Read the model definition and answer for the solid it produces. Units are mm, in the model's axes. Face numbers are marked on the shaded views. A direction names the side the tool comes from. Coordinates: 2 decimals unless noted, no trailing zeros. Order: outer loops, then holes, each group sorted by start corner. A loop starts at its lowest first (then second) coordinate and runs counter-clockwise, first axis right, second up. Notation, with made-up numbers: (1.25, 5.25) -> (52.25, 5.25) arc R8 ccw to (52.25, 18.25) -> close; hole circle Ø8 at (-11.5, 59). An arc over 180 degrees is marked (long way). Answer in a Markdown table with one row per item.
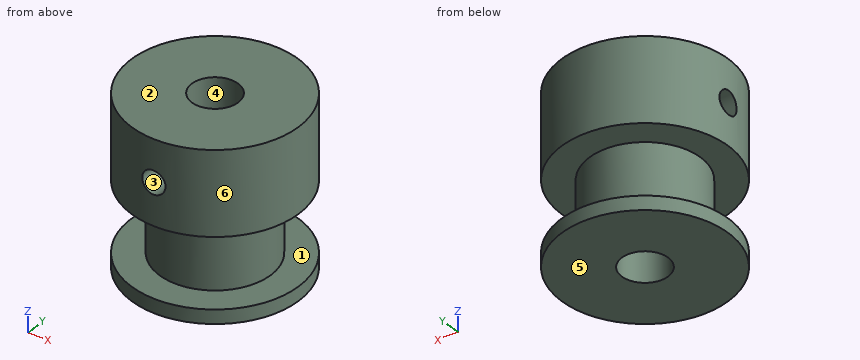
from build123d import *

# Parameters (mm, degrees)
ESQUISSE1_R                  = 9
BOSS_EXTRU_1_DEPTH           = 18
ENL_V_START                  = 1.5
ESQUISSE2_R                  = 9
ESQUISSE2_R_2                = 6
ENL_V_MAT_EXTRU_1_DEPTH      = 7.5
ESQUISSE3_R                  = 2.5
ENL_V_MAT_EXTRU_3_DEPTH      = 23.045407685
ESQUISSE4_R                  = 1.25
ENL_V_MAT_EXTRU_4_DEPTH      = 23.045407685
R_P_TITION_CIRCULAIRE1_COUNT = 2
R_P_TITION_CIRCULAIRE1_ANGLE = 90


with BuildPart() as part:
    # Esquisse1 → Boss.-Extru.1 (new body)
    with BuildSketch(Plane.XY):
        Circle(ESQUISSE1_R)
    extrude(amount=BOSS_EXTRU_1_DEPTH)

    # Esquisse2 → Enlèv. mat.-Extru.1 (cut)
    with BuildSketch(Plane.XY.offset(ENL_V_START)):
        Circle(ESQUISSE2_R)
        Circle(ESQUISSE2_R_2, mode=Mode.SUBTRACT)
    extrude(amount=ENL_V_MAT_EXTRU_1_DEPTH, mode=Mode.SUBTRACT)

    # Esquisse3 → Enlèv. mat.-Extru.3 (cut, through all)
    with BuildSketch(Plane.XY):
        Circle(ESQUISSE3_R)
    extrude(amount=ENL_V_MAT_EXTRU_3_DEPTH, mode=Mode.SUBTRACT)

    # Esquisse4 → Enlèv. mat.-Extru.4 (cut, through all)
    with BuildSketch(Plane(origin=(0, 0, 0), x_dir=(1, 0, 0), z_dir=(0, 1, 0))):
        with Locations(Location((0, -13.5, 0), (0, 0, 270))):
            Circle(ESQUISSE4_R)
    enl_v_mat_extru_4 = extrude(amount=-ENL_V_MAT_EXTRU_4_DEPTH, mode=Mode.SUBTRACT)

    # Répétition circulaire1: Enlèv. mat.-Extru.4 ×2 about axis
    r_p_tition_circulaire1_axis = Axis((0, 0, 18), (0, 0, -1))
    for i in range(1, R_P_TITION_CIRCULAIRE1_COUNT):
        add(enl_v_mat_extru_4.rotate(r_p_tition_circulaire1_axis, i * R_P_TITION_CIRCULAIRE1_ANGLE / (R_P_TITION_CIRCULAIRE1_COUNT - 1)), mode=Mode.SUBTRACT)


solid = part.part
Q1. The part is cut by section D-D (z = 10.5). Write down the section's boundary in (x, y).
Outcome:
| item | result |
|---|---|
| outline | circle Ø18 at (0, 0); hole circle Ø5 at (0, 0) |
Q2. The part is cut by section A-A (x = 0). Write down the section's boundary in (y, z).
Outcome:
| item | result |
|---|---|
| outline | (-9, 0) -> (-2.5, 0) -> (-2.5, 12.25) -> (-9, 12.25) -> (-9, 9) -> (-6, 9) -> (-6, 1.5) -> (-9, 1.5) -> close; (-9, 14.75) -> (-2.5, 14.75) -> (-2.5, 18) -> (-9, 18) -> close; (2.5, 0) -> (9, 0) -> (9, 1.5) -> (6, 1.5) -> (6, 9) -> (9, 9) -> (9, 18) -> (2.5, 18) -> close |
Q3. For the marked faces 1, 2 and 3, determine the directions among +Z, -Z, +X, -X, +Y, -Y from which every point of the face is accessible in a straight line to the end or side of a thin tool.
Outcome:
| item | result |
|---|---|
| face 1 | none |
| face 2 | +Z, +X, -X, +Y, -Y |
| face 3 | -Y |
Q4. For a pull along X with two mould halves and no side action, classify the marked faces 4, 5 and 6 as pulls with the +X half, pulls with the -X half, needs draft (parallel to the pull), parting line crosses it, or undercut.
Outcome:
| item | result |
|---|---|
| face 4 | undercut |
| face 5 | needs draft |
| face 6 | parting line crosses it |
Q5. Given pin 1 (5.5 mm diameter, centred on x = -1.5, y = -2.5, fed in from -Z); pin 2 (6 mm diameter, centred on y = 7, z = 5, fed in from +X); pin 3 (4 mm diameter, centred on x = -5.5, z = 5, fed in from +Y); pin 4 (4 mm diameter, centred on x = 5, z = 6.5, fed in from -Y), each flat-ended and moving along its own axis, determine where each tip first touches the part or whether it passes through.
Outcome:
| item | result |
|---|---|
| pin 1 | z = 0 |
| pin 2 | x = 4.47 |
| pin 3 | y = 4.87 |
| pin 4 | y = -5.2 |
Q6. The part is cut by section B-B (y = -7.25). Write down the section's boundary in (x, z).
Outcome:
| item | result |
|---|---|
| outline | (-5.33, 0) -> (5.33, 0) -> (5.33, 1.5) -> (-5.33, 1.5) -> close; (-5.33, 9) -> (5.33, 9) -> (5.33, 18) -> (-5.33, 18) -> close; hole circle Ø2.5 at (0, 13.5) |
Q7. Consider line 1 (Z direction, x = 8, y = -0.75); line 2 (Z direction, x = 0, y = -7); line 3 (Z direction, x = 0, y = -4.5). Determine where each line is inside the solid, lowest interval first.
Outcome:
| item | result |
|---|---|
| line 1 | 0 to 1.5, 9 to 18 |
| line 2 | 0 to 1.5, 9 to 12.25, 14.75 to 18 |
| line 3 | 0 to 12.25, 14.75 to 18 |
